Geometry check sheet. Reference: the model listing, model coordinates, mm. A direction names the side the tool comes from. Coordinates: 2 decimals unless noted, no trailing zeros. Write each loop counter-clockwise with the first axis right and the second up, starting at its lowest first coordinate (ties: lowest second). Pieces come first, ordered by that corner, then holes.
from build123d import *

# Parameters (mm, degrees)
EXTRUDE_1_DEPTH     = 18
CUT_EXTRUDE_1_REACH = 33.788
CUT_EXTRUDE_2_DEPTH = 6.25
SKETCH_4_R          = 1.0000000000000013
CUT_EXTRUDE_3_DEPTH = 10
SKETCH_8_R          = 3.4999999999999996
SKETCH_8_R_2        = 0.751628678477691
SKETCH_8_R_3        = 0.7516286784776927
EXTRUDE_2_DEPTH     = 2.5
EXTRUDE_3_DEPTH     = 2
CUT_EXTRUDE_4_REACH = 39.597
SKETCH_8_4_R        = 0.751628678477691
SKETCH_8_4_R_2      = 0.7516286784776927


# Read off the part's stored shape, not the designer's step: 凸台-拉伸3
with BuildPart() as part:
    # 草图1 → 凸台-拉伸1 (new, symmetric)
    with BuildSketch(Plane.XY):
        Polygon((0, 0), (0, 10), (-9.5, 9.999999999999998), (-9.499999999999998, 2.5000000000000004), (-11.999999999999998, 2.5), (-17.499999999999996, -3.0000000000000218), (-17.499999999999996, -19.5), (-14.999999999999995, -19.500000000000004), (-14.999999999999995, -4.035533905932752), (-10.964466094067257, -4e-17), align=None)
    extrude(amount=EXTRUDE_1_DEPTH, both=True)

    # 草图2 → 切除-拉伸1 (cut, up to next)
    with BuildSketch(Plane.ZY.offset(17.499999999999996), mode=Mode.PRIVATE) as cut_extrude_1_sk1:
        Polygon((-9.011266099163953, -13.03553390593275), (-11.999999999999996, -13.03553390593275), (-11.999999999999998, -4.035533905932751), (1.5000000000000013, -4.035533905932748), (1.500000000000002, -6.364922727617167), align=None)
    cut_extrude_1_tool1 = extrude(cut_extrude_1_sk1.sketch, amount=-CUT_EXTRUDE_1_REACH, mode=Mode.PRIVATE) & part.part
    # 草图2 → 切除-拉伸1 (cut, up to next)
    with BuildSketch(Plane.ZY.offset(17.499999999999996), mode=Mode.PRIVATE) as cut_extrude_1_sk2:
        Polygon((-7.9999999999999964, -19.499999999999996), (18, -19.49999999999999), (18, -3.000000000000014), align=None)
    cut_extrude_1_tool2 = extrude(cut_extrude_1_sk2.sketch, amount=-CUT_EXTRUDE_1_REACH, mode=Mode.PRIVATE) & part.part
    add(cut_extrude_1_tool1.solids().sort_by_distance((-17.5, -7.612266, -6.566584))[0], mode=Mode.SUBTRACT)
    add(cut_extrude_1_tool2.solids().sort_by_distance((-17.5, -14, 9.333333))[0], mode=Mode.SUBTRACT)

    # 草图3 → 切除-拉伸2 (cut, symmetric)
    with BuildSketch(Plane(origin=(0, 8.89452112858794, -0.8331769279117781), x_dir=(0, -1, 0), z_dir=(1, 0, 0))):
        Polygon((2.3945211285879346, 15.166823072088224), (2.3945211285879346, 10.666823072088222), (8.894521128587936, 10.666823072088222), (8.894521128587936, -12.333176927911778), (2.394521128587931, -12.333176927911778), (2.3945211285879346, -16.833176927911776), (0.8945211285879351, -16.833176927911776), (0.8945211285879351, -12.33317692791178), (-3.1054788714120676, -12.333176927911778), (-3.105478871412064, 10.66682307208822), (0.8945211285879369, 10.66682307208822), (0.8945211285879351, 15.166823072088224), align=None)
    extrude(amount=CUT_EXTRUDE_2_DEPTH, both=True, mode=Mode.SUBTRACT)

    # 草图4 → 切除-拉伸3 (cut)
    with BuildSketch(Plane(origin=(0, 0, 0), x_dir=(0, 0, -1), z_dir=(1, 0, 0))):
        with Locations(Location((-14, 4.500000000000008, 0), (0, 0, 90))):
            Circle(SKETCH_4_R)
    cut_extrude_3 = extrude(amount=-CUT_EXTRUDE_3_DEPTH, mode=Mode.SUBTRACT)

    # 镜向1: 切除-拉伸3 across plane
    add(cut_extrude_3.mirror(Plane.XY), mode=Mode.SUBTRACT)

    # 草图8 → 凸台-拉伸2 (add)
    with BuildSketch(Plane.ZY.offset(17.499999999999996)):
        with BuildLine():
            Line((-20.886363636363633, -11.809802124345238), (-10.090909090909088, -13.295790400552288))
            ThreePointArc((-10.090909090909088, -13.295790400552288), (-7.50000000000001, -16.26776695296638), (-10.090909090909088, -19.239743505380464))
            Line((-10.090909090909088, -19.239743505380464), (-20.886363636363633, -20.725731781587513))
            ThreePointArc((-20.886363636363633, -20.725731781587513), (-25.999999999999996, -16.267766952966376), (-20.886363636363633, -11.809802124345238))
        make_face()
        with Locations(Location((-21.5, -16.267766952966376, 0), (0, 0, 270))):
            Circle(SKETCH_8_R, mode=Mode.SUBTRACT)
        with Locations((-15.499999999999998, -16.267766952966372)):
            Circle(SKETCH_8_R_2, mode=Mode.SUBTRACT)
        with Locations((-10.499999999999998, -16.26776695296638)):
            Circle(SKETCH_8_R_3, mode=Mode.SUBTRACT)
    extrude(amount=-EXTRUDE_2_DEPTH)

    # 凸台-拉伸3 outline → 凸台-拉伸3 (add)
    with BuildSketch(Plane.ZY.offset(17.499999999999996)):
        with BuildLine():
            Line((-11.98162869, -13.035533906), (-12, -13.035533906))
            Line((-12, -13.035533906), (-12, -13.033005105))
            Line((-12, -13.033005105), (-20.886363636, -11.809802124))
            ThreePointArc((-20.886363636, -11.809802124), (-26, -16.267766953), (-20.886363636, -20.725731782))
            Line((-20.886363636, -20.725731782), (-10.090909091, -19.239743505))
            ThreePointArc((-10.090909091, -19.239743505), (-7.5, -16.267766953), (-10.090909091, -13.295790401))
            Line((-10.090909091, -13.295790401), (-11.98162869, -13.035533906))
        make_face()
        with BuildLine():
            ThreePointArc((-21.022727273, -19.735072931), (-25, -16.267766953), (-21.022727273, -12.800460975))
            Line((-21.022727273, -12.800460975), (-10.227272727, -14.286449251))
            ThreePointArc((-10.227272727, -14.286449251), (-8.5, -16.267766953), (-10.227272727, -18.249084655))
            Line((-10.227272727, -18.249084655), (-21.022727273, -19.735072931))
        make_face(mode=Mode.SUBTRACT)
    extrude(amount=EXTRUDE_3_DEPTH)

    # 草图8<4> → 切除-拉伸4 (cut, up to next)
    with BuildSketch(Plane.ZY.offset(17.499999999999996), mode=Mode.PRIVATE) as cut_extrude_4_sk1:
        with Locations(Location((-15.499999999999998, -16.267766952966372, 0), (0, 0, 270))):
            Circle(SKETCH_8_4_R)
    cut_extrude_4_tool1 = extrude(cut_extrude_4_sk1.sketch, amount=-CUT_EXTRUDE_4_REACH, mode=Mode.PRIVATE) & part.part
    # 草图8<4> → 切除-拉伸4 (cut, up to next)
    with BuildSketch(Plane.ZY.offset(17.499999999999996), mode=Mode.PRIVATE) as cut_extrude_4_sk2:
        with Locations(Location((-10.499999999999998, -16.26776695296638, 0), (0, 0, 270))):
            Circle(SKETCH_8_4_R_2)
    cut_extrude_4_tool2 = extrude(cut_extrude_4_sk2.sketch, amount=-CUT_EXTRUDE_4_REACH, mode=Mode.PRIVATE) & part.part
    add(cut_extrude_4_tool1.solids().sort_by_distance((-17.5, -16.267767, -15.5))[0], mode=Mode.SUBTRACT)
    add(cut_extrude_4_tool2.solids().sort_by_distance((-17.5, -16.267767, -10.5))[0], mode=Mode.SUBTRACT)


solid = part.part
1. Sectioned sample at A-A, the plane x = -4.25. Record the boundary of the cut face in (y, z).
Computed values:
outline: (0, -18) - (10, -18) - (10, -11.5) - (8, -11.5) - (8, -16) - (6.5, -16) - (6.5, -11.5) - (0, -11.5) - close; (0, 11.5) - (6.5, 11.5) - (6.5, 16) - (8, 16) - (8, 11.5) - (10, 11.5) - (10, 18) - (0, 18) - close; hole circle Ø2 at (4.5, -14); hole circle Ø2 at (4.5, 14)
2. Thickness scan on line 1 along Y through (x, z) = (-3.5, -14); line 2 along Y through (x, z) = (-18.4, -21.5); line 3 along Z through (x, y) = (-12.75, 1.5). Record the ranges inside material, lowest first.
Computed values:
line 1: y = 0 to 3.5, 5.5 to 6.5, 8 to 10
line 2: y = -20.77 to -19.77, -12.77 to -11.77
line 3: z = -18 to 18
3. Sectioned sample at C-C, the plane z = -21.5. Record the boundary of the cut face in (x, y), and give its area (3 significant figures).
Computed values:
outline: (-19.5, -20.77) - (-15, -20.77) - (-15, -19.77) - (-19.5, -19.77) - close; (-19.5, -12.77) - (-15, -12.77) - (-15, -11.77) - (-19.5, -11.77) - close
area: 9.00 mm2
4. Sectioned sample at D-D, the plane x = -8. Record the boundary of the cut face in (y, z), and give its area (3 significant figures).
Computed values:
outline: (0, -18) - (10, -18) - (10, 18) - (0, 18) - close; hole circle Ø2 at (4.5, -14); hole circle Ø2 at (4.5, 14)
area: 354 mm2
5. Gauge pin test, flat ends, axial feed: pin 1 Ø1.5 at (x, y) = (-16.5, -1.5) entering from -Z; pin 2 Ø11 at (y, z) = (-16.27, -21.5) entering from -X; pin 3 Ø13 at (y, z) = (-8, 0) entering from -X; pin 4 Ø1.3 at (x, z) = (-4, 14.5) entering from -Y. Record the tip position at first contact, or that the pin passes through.
Computed values:
pin 1: stops at z = -18
pin 2: stops at x = -19.5
pin 3: stops at x = -17.5
pin 4: stops at y = 0
6. Access from +Z, -Z, +X, -X, +Y, -Y to the whole of each face (thin tool, end or side, straight path). Record for faces 4 (the flat face through (-16, -13.036, -10)), 5 (the flat face through (-18.486, -13.533, -15.701)), 6 (the flat face through (-9.5, 6, 0)), 7 (the flat face through (-15, -12, -5)), 8 (the flat face through (-16, -19.5, -10)).
Computed values:
face 4: +X, -X
face 5: -X
face 6: +Z, -Z, -X, +Y
face 7: +Z, -Z, +X, -Y
face 8: +Z, +X, -X, -Y
7. Draft check along Y on faces 1 (the flat face through (-3, 9, 11.5)), 2 (the flat face through (-18.486, -13.167, -11.023)), 3 (the flat face through (-3, 6.5, 14)). Enter one of: released by +Y, released by -Y, zero draft, split by the parting line, or undercut.
Computed values:
face 1: zero draft
face 2: released by +Y
face 3: undercut
8. Sectioned sample at B-B, the plane y = 4.5. Record the boundary of the cut face in (x, z).
Computed values:
outline: (-9.5, -18) - (0, -18) - (0, -15) - (-9.5, -15) - close; (-9.5, -13) - (0, -13) - (0, -11.5) - (-6.25, -11.5) - (-6.25, 11.5) - (0, 11.5) - (0, 13) - (-9.5, 13) - close; (-9.5, 15) - (0, 15) - (0, 18) - (-9.5, 18) - close
